For this review, use the dimensioned drawing (mm, ordinates from the lowest corner) and the shaded views. A direction names the side the tool comes from. Give positions to 0.01 mm unless a question says otherwise; leave off trailing zeros. Order: outer loops, then holes, each group sorted by start corner. A loop starts at its lowest first (then second) coordinate and runs counter-clockwise, first axis right, second up.
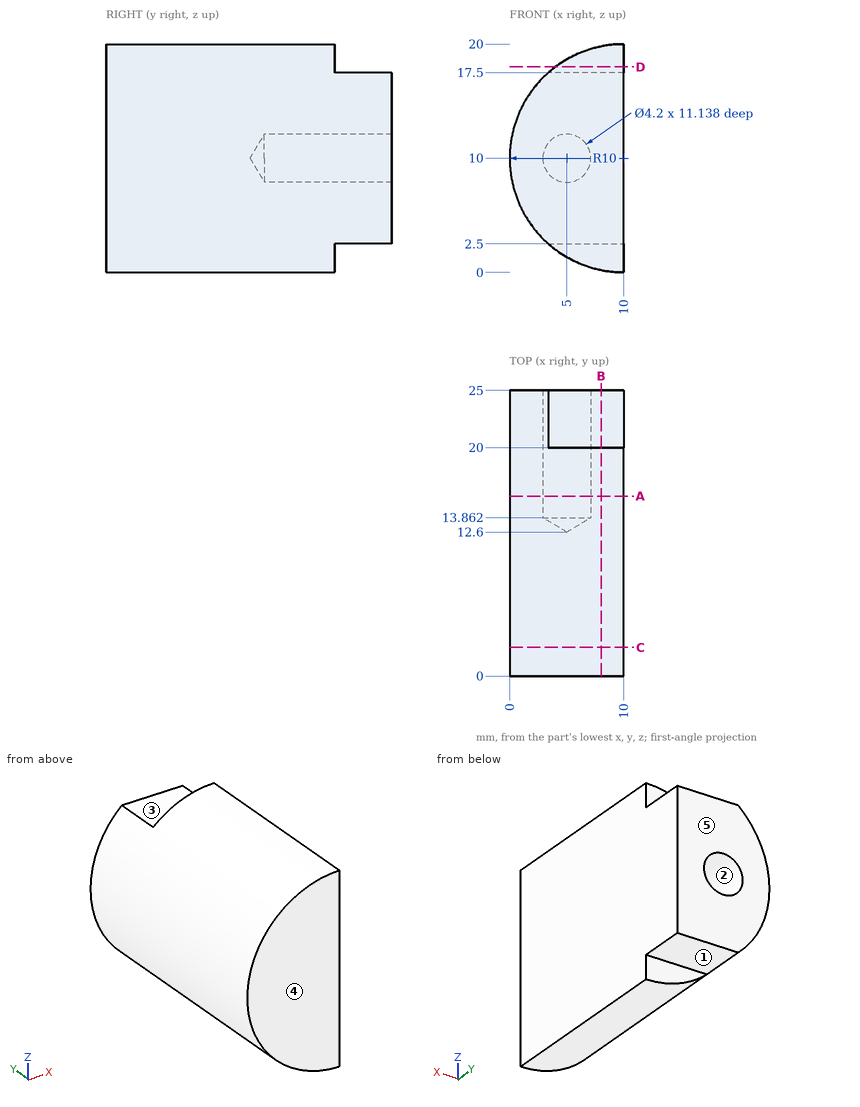
1. For line 1 along X through (y, z) = (17.5, 10); line 2 along Y through (x, z) = (8.5, 19); line 3 along Z through (x, y) = (5, 16), list the stretches that pass through material, from the lowest coordinate up.
Recorded:
line 1: x = 0 to 2.9, 7.1 to 10
line 2: y = 0 to 20
line 3: z = 1.34 to 7.9, 12.1 to 18.66
2. For pin 1 (3 mm diameter, centred on x = 1.5, y = 16, fed in from +Z); pin 2 (1.2 mm diameter, centred on x = 6, z = 2, fed in from +Y); pin 3 (1.5 mm diameter, centred on x = 7, y = 21.5, fed in from -Z); pin 4 (5 mm diameter, centred on x = 1.5, y = 18, fed in from -Z), all flat-tipped, find the tip position at first contact; note any pin that passes through.
Recorded:
pin 1: stops at z = 17.14
pin 2: stops at y = 25
pin 3: stops at z = 2.5
pin 4: stops at z = 2
3. Take a section at C-C (y = 2.5). State the section outline as (x, z) points.
Recorded:
outline: (10, 0) - (10, 20) arc R10 ccw to start
4. Machinability: for the marked faces 1, 2, 3, 4 and 5, which of the approach directions +Z, -Z, +X, -X, +Y, -Y give a long, thin tool a straight path to every point of the face, cutting with its end or side? Answer none if there is none.
Recorded:
face 1: -Z, +X, -X, +Y
face 2: +Y
face 3: +Z, +X, -X, +Y
face 4: +Z, -Z, +X, -X, -Y
face 5: +Z, -Z, +X, -X, +Y
5. Take a section at D-D (z = 18). State the section outline as (x, y) points, then the cut area to 3 significant figures.
Recorded:
outline: (4, 0) - (10, 0) - (10, 20) - (4, 20) - close
area: 120 mm2
6. Take a section at B-B (x = 8). State the section outline as (y, z) points.
Recorded:
outline: (0, 0.2) - (20, 0.2) - (20, 2.5) - (25, 2.5) - (25, 17.5) - (20, 17.5) - (20, 19.8) - (0, 19.8) - close
7. Take a section at A-A (y = 15.75). State the section outline as (x, z) points, then the cut area to 3 significant figures.
Recorded:
outline: (10, 0) - (10, 20) arc R10 ccw to start; hole circle Ø4.2 at (5, 10)
area: 143 mm2
